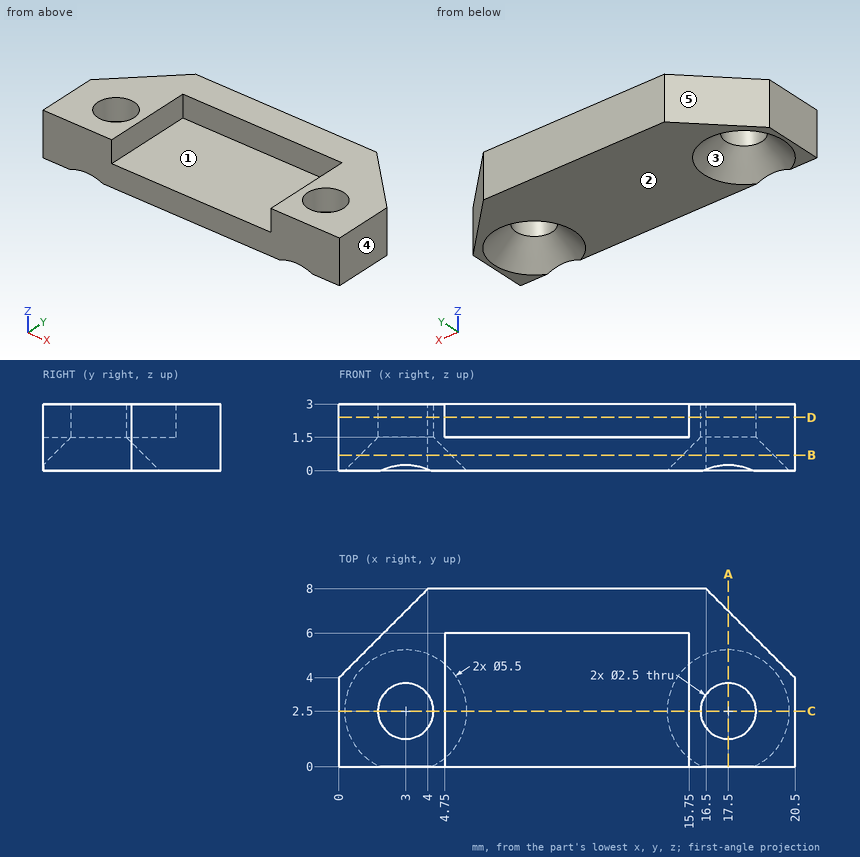
Drawing for the job (mm, zero at the part's lowest x, y, z). A direction names the side the tool comes from. Round coordinates to 2 decimals unless told otherwise and drop trailing zeros. Loops run counter-clockwise (first coordinate to the right, second up) from the corner with the lowest first, then second, coordinate; pieces in that order, holes last. Notation, with made-up numbers: (1.5, 55.25) -> (9.5, 55.25) arc R13 ccw to (9.5, 65.25) -> close; hole circle Ø4 at (-1.5, -19.5). An arc over 180 degrees is marked (long way). Answer in a Markdown table with one row per item.
Item 1: Which spindle directions (+Z, -Z, +X, -X, +Y, -Y) get a long thin tool onto all of the face, cutting with end or side? Do the marked faces 1 and 2. Say none if no direction does.
Answers below:
| item | result |
|---|---|
| face 1 | +Z, -Y |
| face 2 | -Z, +X, -X, +Y, -Y |
Item 2: Pin check, flat tips, straight feed: pin 1 (1 mm diameter, centred on x = 9.5, z = 1.5, fed in from -Y); pin 2 (3 mm diameter, centred on x = 3, y = 2.5, fed in from -Z); pin 3 (2 mm diameter, centred on x = 17.5, y = 2.5, fed in from +Z); pin 4 (3 mm diameter, centred on x = 10.5, y = 3, fed in from +Z). Stop position of each tip, or through.
Answers below:
| item | result |
|---|---|
| pin 1 | stops at y = 0 |
| pin 2 | stops at z = 1.25 |
| pin 3 | passes through |
| pin 4 | stops at z = 1.5 |
Item 3: Saw through at D-D (z = 2.4). Write the cut outline in (x, y).
Answers below:
| item | result |
|---|---|
| outline | (0, 0) -> (4.75, 0) -> (4.75, 6) -> (15.75, 6) -> (15.75, 0) -> (20.5, 0) -> (20.5, 4) -> (16.5, 8) -> (4, 8) -> (0, 4) -> close; hole circle Ø2.5 at (3, 2.5); hole circle Ø2.5 at (17.5, 2.5) |
Item 4: Saw through at B-B (z = 0.7). Write the cut outline in (x, y), and give its area (3 significant figures).
Answers below:
| item | result |
|---|---|
| outline | (0, 0) -> (20.5, 0) -> (20.5, 4) -> (16.5, 8) -> (4, 8) -> (0, 4) -> close; hole circle Ø4.1 at (3, 2.5); hole circle Ø4.1 at (17.5, 2.5) |
| area | 122 mm² |
Item 5: Drill centre lines: L1, parallel to X at y = 3.25, z = 1.3; L2, parallel to X at y = 1.75, z = 1.8; L3, parallel to X at y = 0.5, z = 2.8. Where is each one in solid material? Low to high. Write a range as [from, to].
Answers below:
| item | result |
|---|---|
| L1 | x = [0, 1.76], [4.24, 16.26], [18.74, 20.5] |
| L2 | x = [0, 2], [4, 4.75], [15.75, 16.5], [18.5, 20.5] |
| L3 | x = [0, 4.75], [15.75, 20.5] |
Item 6: Saw through at C-C (y = 2.5). Write the cut outline in (x, z), and give its area (3 significant figures).
Answers below:
| item | result |
|---|---|
| outline | (0, 0) -> (0.25, 0) -> (1.75, 1.5) -> (1.75, 3) -> (0, 3) -> close; (4.25, 1.5) -> (5.75, 0) -> (14.75, 0) -> (16.25, 1.5) -> (16.25, 3) -> (15.75, 3) -> (15.75, 1.5) -> (4.75, 1.5) -> (4.75, 3) -> (4.25, 3) -> close; (18.75, 1.5) -> (20.25, 0) -> (20.5, 0) -> (20.5, 3) -> (18.75, 3) -> close |
| area | 25.5 mm² |
Item 7: Mould opens along Y. For the marked faces 3, 4 and 5 say: +Y half, -Y half, draft (parallel to the pull), parting line (faces both ways), or undercut.
Answers below:
| item | result |
|---|---|
| face 3 | undercut |
| face 4 | draft |
| face 5 | +Y half |
Item 8: Saw through at A-A (x = 17.5). Write the cut outline in (y, z), and give its area (3 significant figures).
Answers below:
| item | result |
|---|---|
| outline | (0, 0.25) -> (1.25, 1.5) -> (1.25, 3) -> (0, 3) -> close; (3.75, 1.5) -> (5.25, 0) -> (7, 0) -> (7, 3) -> (3.75, 3) -> close |
| area | 11.3 mm² |
